Solid Edge part; units mm, degrees
sketch "Sketch1" plane through (0, 0, 0) normal (1, 0, 0) x (0, 1, 0)
  line L0 (8, 34) -> (8, 50)
  line L1 (0, 50) -> (8, 50)
  line L2 (0, 50) -> (0, 34)
  line L3 (0, 34) -> (-5, 34)
  line L4 (-5, 34) -> (-5, 29)
  line L5 (-5, 29) -> (0, 29)
  line L6 (0, 29) -> (0, 23.5)
  line L7 (0, 23.5) -> (4, 23.5)
  line L8 (4, 23.5) -> (4, 26)
  line L9 (4, 26) -> (11, 26)
  line L10 (11, 34) -> (11, 26)
  line L11 (11, 34) -> (8, 34)
revolve "RevolvedProtrusion1" add sketch "Sketch1" angle 360 about axis through (0, -22.1591, 0) along (0, 1, 0)
hole "Hole1" at (29.6985, 8, 29.6985) direction (0, -1, 0) diameter 8.5 end through all
hole "Hole2" at (-29.6985, 8, 29.6985) direction (0, -1, 0) diameter 8.5 end through all
hole "Hole3" at (-29.6985, 8, -29.6985) direction (0, -1, 0) diameter 8.5 end through all
hole "Hole4" at (29.6985, 8, -29.6985) direction (0, -1, 0) diameter 8.5 end through all
Check sheet for the modelled part. Datum: model origin and axes. Units: mm. A direction names the side the tool comes from. Coordinates: 2 decimals unless noted, no trailing zeros. Write each loop counter-clockwise with the first axis right and the second up, starting at its lowest first coordinate (ties: lowest second). Pieces come first, ordered by that corner, then holes. Notation, with made-up numbers: M 43,67.25 L 54,67.25 A15 ccw 54,93.25 Z; hole C 80.25,77 d11. An arc over 180 degrees is marked long. Use one line per item in the form item = value.
Item 1: Sectioned sample at A-A, the plane z = 0. Record the cut outline in (x, y).
Answer below:
outline = M -50,0 L -34,0 L -34,-5 L -29,-5 L -29,0 L -23.5,0 L -23.5,4 L -26,4 L -26,11 L -34,11 L -34,8 L -50,8 Z; M 23.5,0 L 29,0 L 29,-5 L 34,-5 L 34,0 L 50,0 L 50,8 L 34,8 L 34,11 L 26,11 L 26,4 L 23.5,4 Z
Item 2: Material ranges on L1, parallel to Z at x = -29, y = 6; L2, parallel to X at y = 6.75, z = 0; L3, parallel to X at y = 2.9, z = 0, recorded low to high. Write a range as from..to.
Answer below:
L1 = -40.73..-33.89, -25.51..25.51, 33.89..40.73
L2 = -50..-26, 26..50
L3 = -50..-23.5, 23.5..50
Item 3: Sectioned sample at D-D, the plane z = 38.5. Record the cut outline in (x, y), and give its area (3 significant figures).
Answer below:
outline = M -31.9,0 L 31.9,0 L 31.9,8 L -31.9,8 Z
area = 510 mm^2
Item 4: Sectioned sample at C-C, the plane y = -2.5. Record the cut outline in (x, z).
Answer below:
outline = C 0,0 d68; hole C 0,0 d58
Item 5: Set-up check for faces 1 (the face through (-25, 11, -8)), 2 (the face through (-33, 8, 10)), 3 (the face through (-25.73, -2.46, 13.38)): record each of +Z, -Z, +X, -X, +Y, -Y from which the full face is reachable in a straight line by a thin tool's end or side.
Answer below:
face_1 = +Z, -Z, +X, -X, +Y
face_2 = +Y
face_3 = -Y
Item 6: Release check for a two-part mould opening along Z. For faces 4 (the face through (-28.67, 9.48, 18.28)), 5 (the face through (-15.821, 7.549, -20.633)), 6 (the face through (-33, 0, 10)), 7 (the face through (-23, 4, -6)) record: pulls with the +Z half, pulls with the -Z half, needs draft (parallel to the pull), parting line crosses it, or undercut.
Answer below:
face_4 = parting line crosses it
face_5 = undercut
face_6 = needs draft
face_7 = undercut
Item 7: Sectioned sample at B-B, the plane x = 0. Record the cut outline in (y, z).
Answer below:
outline = M -5,-34 L 0,-34 L 0,-50 L 8,-50 L 8,-34 L 11,-34 L 11,-26 L 4,-26 L 4,-23.5 L 0,-23.5 L 0,-29 L -5,-29 Z; M -5,29 L 0,29 L 0,23.5 L 4,23.5 L 4,26 L 11,26 L 11,34 L 8,34 L 8,50 L 0,50 L 0,34 L -5,34 Z
Item 8: Gauge pin test, flat ends, axial feed: pin 1 Ø2 at (x, z) = (14.5, 35.5) entering from -Y; pin 2 Ø8 at (y, z) = (-1, 14.5) entering from -X; pin 3 Ø5 at (y, z) = (-1, 10.5) entering from +X. Record the tip position at first contact, or that the pin passes through.
Answer below:
pin_1 = 0
pin_2 = -48.86
pin_3 = 49.32
